CAD build for the part. Positions are in the model's coordinates, mm. A direction names the side the tool comes from. Coordinates: 2 decimals unless noted, no trailing zeros. Loops run counter-clockwise (first coordinate to the right, second up) from the corner with the lowest first, then second, coordinate; pieces in that order, holes last. Notation, with made-up numbers: (32.25, 18) -> (43.25, 18) arc R27 ccw to (43.25, 45) -> close; hole circle Ø2 at (-7.5, 14). An arc over 180 degrees is marked (long way). Return JSON: item names as keys, results as strings. Group by question number.
(1) Probe L1, parallel to Y at x = 1.1, z = -1.9; L2, parallel to Y at x = 2.65, z = -1.1; L3, parallel to Z at x = -0.3, y = 22. List the from-to ranges inside material, lowest first.
(2) Flat gauge pins, fed straight in: pin 1 Ø3 at (x, y) = (-2, 11.5) entering from +Z; pin 2 Ø1.5 at (y, z) = (6, 1) entering from +X. Where does each tip first touch, or does it go through?
(3) Saw through at A-A on z = 0. Write the cut outline in (x, y), then the cut area to 3 significant figures.
(4) Saw through at C-C on y = 16.75. Write the cut outline in (x, z), then the cut area to 3 significant figures.
(5) Saw through at B-B on x = 0. Write the cut outline in (y, z).
(6) Tool access for faces 1 (the face through (-1, 28.06, 2)), 2 (the face through (0, 30, 0)): list every direction of +Z, -Z, +X, -X, +Y, -Y with a clear straight run to the whole face (end or side of a thin tool).
```python
from build123d import *

# Parameters (mm, degrees)
SKETCH1_R           = 3
BOSS_EXTRUDE1_DEPTH = 30
SKETCH2_W           = 1
SKETCH2_H           = 0.74
CHAMFER1_SIZE       = 0.5


with BuildPart() as part:
    # Sketch1 → Boss-Extrude1 (new body)
    with BuildSketch(Plane(origin=(0, 0, 0), x_dir=(1, 0, 0), z_dir=(0, 1, 0))):
        with Locations(Location((0, 0, 0), (0, 0, 270))):
            Circle(SKETCH1_R)
    extrude(amount=BOSS_EXTRUDE1_DEPTH)

    # Sketch2 → Cut-Revolve1 (revolve, cut)
    with BuildSketch(Plane.XY):
        with Locations((2.5, 28.43)):
            Rectangle(SKETCH2_W, SKETCH2_H)
        with Locations((2.5, 1.57)):
            Rectangle(SKETCH2_W, SKETCH2_H)
    revolve(axis=Axis((0, -1000, 0), (0, 1, 0)), mode=Mode.SUBTRACT)

    # Chamfer1
    chamfer1_edges = [part.edges().sort_by_distance(p)[0] for p in [
        (0, 0, -3),
        (0, 30, -3),
    ]]
    chamfer(chamfer1_edges, length=CHAMFER1_SIZE)


solid = part.part
```
Geometry results:
{
 "1": {"L1": "0 to 1.2, 1.94 to 28.06, 28.8 to 30", "L2": "0.37 to 1.2, 1.94 to 28.06, 28.8 to 29.63", "L3": "-2.98 to 2.98"},
 "2": {"pin 1": "z = 2.96", "pin 2": "x = 2.99"},
 "3": {"outline": "(-3, 0.5) -> (-2.5, 0) -> (2.5, 0) -> (3, 0.5) -> (3, 1.2) -> (2, 1.2) -> (2, 1.94) -> (3, 1.94) -> (3, 28.06) -> (2, 28.06) -> (2, 28.8) -> (3, 28.8) -> (3, 29.5) -> (2.5, 30) -> (-2.5, 30) -> (-3, 29.5) -> (-3, 28.8) -> (-2, 28.8) -> (-2, 28.06) -> (-3, 28.06) -> (-3, 1.94) -> (-2, 1.94) -> (-2, 1.2) -> (-3, 1.2) -> close", "area": "177 mm²"},
 "4": {"outline": "circle Ø6 at (0, 0)", "area": "28.3 mm²"},
 "5": {"outline": "(0, -2.5) -> (0.5, -3) -> (1.2, -3) -> (1.2, -2) -> (1.94, -2) -> (1.94, -3) -> (28.06, -3) -> (28.06, -2) -> (28.8, -2) -> (28.8, -3) -> (29.5, -3) -> (30, -2.5) -> (30, 2.5) -> (29.5, 3) -> (28.8, 3) -> (28.8, 2) -> (28.06, 2) -> (28.06, 3) -> (1.94, 3) -> (1.94, 2) -> (1.2, 2) -> (1.2, 3) -> (0.5, 3) -> (0, 2.5) -> close"},
 "6": {"face 1": "none", "face 2": "+Z, -Z, +X, -X, +Y"}
}
